The figure shows three views and two pictorial views of one solid part (mm, origin at its lowest corner). Answer the questions. A direction names the side the tool comes from. Coordinates: 2 decimals unless noted, no trailing zeros. Order: outer loops, then holes, each group sorted by start corner. A loop starts at its lowest first (then second) coordinate and runs counter-clockwise, first axis right, second up.
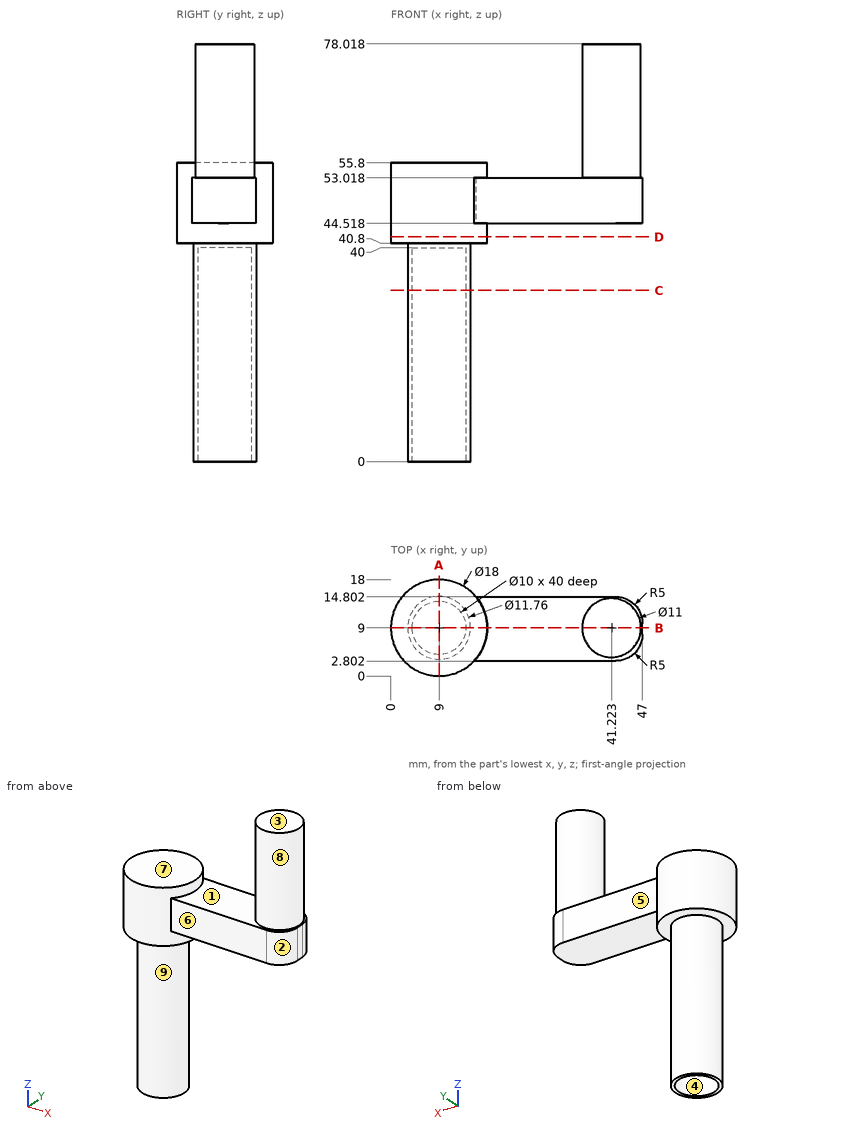
1) The mould has two halves that part along X. Classify the marked faces 1, 2, 3 and 4: released by +X, released by -X, zero draft, split by the parting line, or undercut.
2) Each of these flat-tipped pins is pushed along its axis until it touches: P1, Ø5, axis at x = 11, y = 10, coming from the -Z side; P2, Ø10, axis at x = 19.5, y = 14.5, coming from the +Z side; P3, Ø1.5, axis at x = 22, y = 5, coming from the +Z side; P4, Ø9, axis at x = 7.5, y = 13.5, coming from the -Z side. Where does it stop, or does it pass through?
3) A cutting plane is placed at B-B, the plane y = 9. Write down the section's boundary in (x, z).
4) For the marked faces 5, 6, 7, 8 and 9, determine the directions among +Z, -Z, +X, -X, +Y, -Y from which every point of the face is accessible in a straight line to the end or side of a thin tool.
5) A cutting plane is placed at C-C, the plane z = 32. Write down the section's boundary in (x, y).
6) A cutting plane is placed at A-A, the plane x = 9. Write down the section's boundary in (y, z).
7) Straight lines are drawn through the part: probe 1 along Y at (x, z) = (9, 25); probe 2 along Z at (x, y) = (45, 7); probe 3 along Z at (x, y) = (5, 1). For each, find the intervals that lie inside material, in ascending order.
8) A cutting plane is placed at D-D, the plane z = 42. Write down the section's boundary in (x, y).
Working result:
1. face 1: undercut
1. face 2: released by +X
1. face 3: zero draft
1. face 4: undercut
2. P1: stops at z = 40
2. P2: stops at z = 55.8
2. P3: stops at z = 53.02
2. P4: stops at z = 0
3. outline: (0, 40.8) - (3.12, 40.8) - (3.12, 0) - (4, 0) - (4, 40) - (14, 40) - (14, 0) - (14.88, 0) - (14.88, 40.8) - (18, 40.8) - (18, 44.52) - (47, 44.52) - (47, 53.02) - (46.72, 53.02) - (46.72, 78.02) - (35.72, 78.02) - (35.72, 53.02) - (18, 53.02) - (18, 55.8) - (0, 55.8) - close
4. face 5: +Z, -Z, +X, +Y
4. face 6: +Z, -Z, +X, -Y
4. face 7: +Z, -X, +Y, -Y
4. face 8: +Z
4. face 9: -Z
5. outline: circle Ø11.76 at (9, 9); hole circle Ø10 at (9, 9)
6. outline: (0, 40.8) - (3.12, 40.8) - (3.12, 0) - (4, 0) - (4, 40) - (14, 40) - (14, 0) - (14.88, 0) - (14.88, 40.8) - (18, 40.8) - (18, 55.8) - (0, 55.8) - close
7. probe 1: y = 3.12 to 4, 14 to 14.88
7. probe 2: z = 44.52 to 78.02
7. probe 3: z = 40.8 to 55.8
8. outline: circle Ø18 at (9, 9)
